Could you check a few things on this model? Use its own coordinates, in mm. Face numbers are marked on the shaded views. A direction names the side the tool comes from. Give positions to 0.01 mm unless a question says otherwise; leave off trailing zeros. Order: outer loops, then holes, each group sorted by start corner. A loop starts at its lowest first (then second) coordinate and runs counter-clockwise, first axis right, second up. Notation, with made-up numbers: (51.25, 16) - (104.25, 16) arc R17 cw to (104.25, 40) - close; hole circle Ø11 at (68.25, 41). An arc over 180 degrees is marked (long way). One line per question, with ' | ' between items. Start each with the question number.
1. Imagine slicing it at A-A (y = 7). Please give me the cut outline in (x, z).
2. Which directions (+Z, -Z, +X, -X, +Y, -Y) give clear straight access to the entire face, cutting with the end or side of a thin tool? Please do the marked faces 4, 5 and 6.
3. If we mould it in two halves opening along X, with no side actions, what happens to the marked faces 1, 2 and 3? For each: released by +X, released by -X, zero draft, split by the parting line, or undercut.
4. For P1, Ø0.5, axis at x = 0, z = 2.5, coming from the +Y side; P2, Ø1, axis at x = 2.5, z = 4.5, coming from the -Y side, each with a flat end and sliding along its axis, tell me the tip position at first contact or that it passes through.
5. I need wall thicknesses on probe 1 along Z at (x, y) = (0, -1); probe 2 along Z at (x, y) = (-2, 6.5); probe 3 along X at (y, z) = (5.5, 3.5). Which ranges of each line are inside material? Lowest first, please. Write a range as from..to.
6. Imagine slicing it at D-D (y = -2.75). Please give me the cut outline in (x, z).
7. Imagine slicing it at B-B (x = -1.5). Please give me the cut outline in (y, z).
8. Imagine slicing it at C-C (z = -3.75). Please give me the cut outline in (x, y), and give its area (3 significant figures).
Autodesk Inventor part; units mm, degrees
ref_plane "YZ Plane" through (0, 0, 0) normal (1, 0, 0) x (0, 1, 0)
ref_plane "XZ Plane" through (0, 0, 0) normal (0, 1, 0) x (-1, 0, 0)
ref_plane "XY Plane" through (0, 0, 0) normal (0, 0, 1) x (1, 0, 0)
sketch "Sketch1" plane through (0, 0, 0) normal (0, 1, 0) x (-1, 0, 0)
  line L0 (4.25, 11.62) -> (-4.25, 11.62)
  line L1 (-4.25, 11.62) -> (-4.25, -11.62)
  line L2 (-4.25, -11.62) -> (4.25, -11.62)
  line L3 (4.25, -11.62) -> (4.25, 11.62)
  point P0 (0, 0)
  dimension "d0" = 23.24
  dimension "d1" = 11.62
  dimension "d2" = 8.5
  dimension "d3" = 4.25
extrude "Extrusion1" add sketch "Sketch1" along normal blind 9.53
fillet "Fillet1" radius 2 4 edges at (4.25, 4.765, 11.62) (-4.25, 4.765, 11.62) (-4.25, 4.765, -11.62) (4.25, 4.765, -11.62)
sketch "Sketch2" plane through (0, 9.53, 0) normal (0, 1, 0) x (1, 0, 0)
  line L0 (-3.25, -10.62) -> (3.25, -10.62)
  line L1 (3.25, -10.62) -> (3.25, 10.62)
  line L2 (3.25, 10.62) -> (-3.25, 10.62)
  line L3 (-3.25, 10.62) -> (-3.25, -10.62)
  line L4 (4.25, 11.62) -> (-4.25, 11.62)
  line L5 (-4.25, 11.62) -> (-4.25, -11.62)
  line L6 (-4.25, -11.62) -> (4.25, -11.62)
  line L7 (4.25, -11.62) -> (4.25, 11.62)
  line L8 (1.25, 10.62) -> (3.25, 8.62)
  line L9 (3.25, -8.62) -> (1.25, -10.62)
  point P0 (0, 0)
  dimension "d6" = 1
  dimension "d7" = 1
  dimension "d8" = 1
  dimension "d9" = 1
  dimension "d11" = 45
  dimension "d12" = 45
  dimension "d13" = 2
  dimension "d14" = 2
extrude "Extrusion2" cut sketch "Sketch2" against normal blind 5.08 contours L3 L2 L8 L1 L9 L0
sketch "Sketch3" plane through (0, 0, 0) normal (0, -1, 0) x (1, 0, 0)
  circle A0 centre (0, 7.62) radius 0.8
  point P0 (0, 0)
  dimension "d17" = 1.6
  dimension "d18" = 7.62
extrude "Extrusion3" add sketch "Sketch3" along normal blind 4.57 and the other way blind 8.89
fillet "Fillet2" radius 0.508 1 edges at (-0.8, 8.89, 7.62)
chamfer "Chamfer1" distance 1 angle 15 1 edges at (-0.8, -4.57, 7.62) measured on face at (0.7974, -3.0467, 7.5556)
pattern_linear "Rectangular Pattern1" count 4 spacing 5.08 along (0, 0, -1) of "Extrusion3", "Fillet2", "Chamfer1"
properties part number "Molex_4x508_Conn"
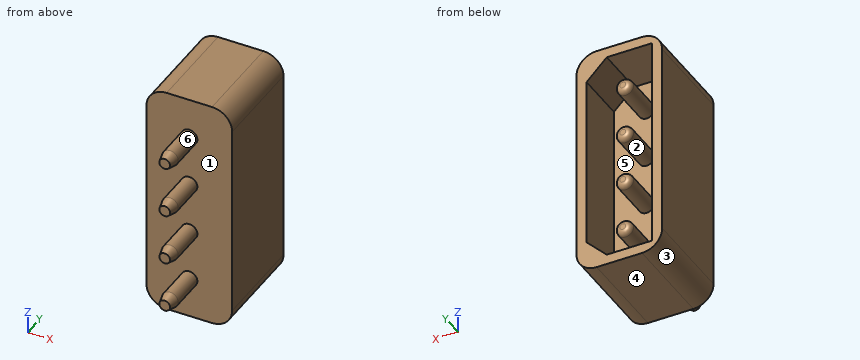
Results found:
1) outline: (-4.25, -9.62) arc R2 ccw to (-2.25, -11.62) - (2.25, -11.62) arc R2 ccw to (4.25, -9.62) - (4.25, 9.62) arc R2 ccw to (2.25, 11.62) - (-2.25, 11.62) arc R2 ccw to (-4.25, 9.62) - close; circle Ø1.6 at (0, -7.62); circle Ø1.6 at (0, -2.54); circle Ø1.6 at (0, 2.54); circle Ø1.6 at (0, 7.62); hole (-3.25, -10.62) - (1.25, -10.62) - (3.25, -8.62) - (3.25, 8.62) - (1.25, 10.62) - (-3.25, 10.62) - close
2) face 4: -Z, +X, -X, +Y, -Y | face 5: +Y | face 6: -Y
3) face 1: zero draft | face 2: undercut | face 3: released by -X
4) P1: stops at y = 8.89 | P2: stops at y = 0
5) probe 1: z = -8.42..-6.82, -3.34..-1.74, 1.74..3.34, 6.82..8.42 | probe 2: z = -11.62..-10.62, 10.62..11.62 | probe 3: x = -4.25..-3.25, 3.25..4.25
6) outline: circle Ø1.6 at (0, -7.62); circle Ø1.6 at (0, -2.54); circle Ø1.6 at (0, 2.54); circle Ø1.6 at (0, 7.62)
7) outline: (0, -11.62) - (9.53, -11.62) - (9.53, -10.62) - (4.45, -10.62) - (4.45, 10.62) - (9.53, 10.62) - (9.53, 11.62) - (0, 11.62) - close
8) outline: (-4.25, 0) - (4.25, 0) - (4.25, 9.53) - (3.25, 9.53) - (3.25, 4.45) - (-3.25, 4.45) - (-3.25, 9.53) - (-4.25, 9.53) - close | area: 48.0 mm2
